Input: part model. Units: mm. Frame: model coordinates. Round coordinates to 2 decimals unless told otherwise and drop trailing zeros. Order: outer loops, then holes, each group sorted by start corner. A loop starts at its lowest first (then second) coordinate and runs counter-clockwise, first axis right, second up. Notation, with made-up numbers: (0.25, 64.25) - (9.25, 64.25) arc R11 ccw to (9.25, 80.25) - close; hole circle Ø4 at (79, 1.5). An arc over 180 degrees is marked (long way). One line per item, written item: value. Start each with the question number.
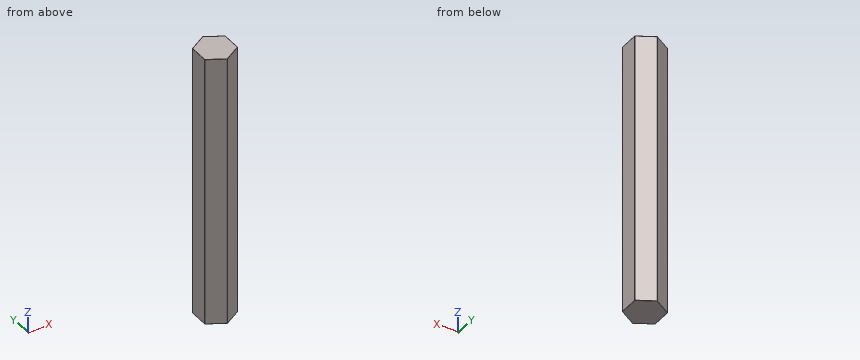
from build123d import *

# Parameters (mm, degrees)
F1_DEPTH = 200
F2_R     = 0.2


with BuildPart() as f1:
    # F0 (on Top) → F1 (new body)
    with BuildSketch(Plane.XY):
        Polygon((-0.015583, -13.856398), (11.992201, -6.941694), (12.007784, 6.914704), (0.015583, 13.856398), (-11.992201, 6.941694), (-12.007784, -6.914704), align=None)
    extrude(amount=F1_DEPTH)

    # F2
    f2_edges = [f1.edges().sort_by_distance(p)[0] for p in [
        (5.988309, -10.399046, 200),
        (11.999992, -0.013495, 200),
        (6.011683, 10.385551, 200),
        (-5.988309, 10.399046, 200),
        (-11.999992, 0.013495, 200),
        (-6.011683, -10.385551, 200),
        (11.992201, -6.941694, 100),
        (12.007784, 6.914704, 100),
        (11.999992, -0.013495, 0),
        (0.015583, 13.856398, 100),
        (6.011683, 10.385551, 0),
        (-11.992201, 6.941694, 100),
        (-5.988309, 10.399046, 0),
        (-12.007784, -6.914704, 100),
        (-11.999992, 0.013495, 0),
        (-0.015583, -13.856398, 100),
        (-6.011683, -10.385551, 0),
    ]]
    fillet(f2_edges, radius=F2_R)


solid = f1.part
Item 1: Line query: L1, parallel to X at y = -4.75, z = 93; L2, parallel to Y at x = 3.5, z = 164.5; L3, parallel to Y at x = 3.25, z = 119.5. Output: solid intervals per line, ascending.
Item 2: First-contact query: pin 1 Ø2 at (x, z) = (-5, 131) entering from +Y; pin 2 Ø4 at (x, z) = (-1.5, 29.5) entering from -Y; pin 3 Ø6 at (x, z) = (5, 135) entering from -Y; pin 4 Ø1 at (y, z) = (7, 103.5) entering from -X. Flat tips, straight axial feed; report the tip coordinate or a pass-through.
Item 3: Section query A-A on z = 119. Return loops of the section in (x, y).
Geometry results:
1. L1: x = -12.01 to 11.99
1. L2: y = -11.83 to 11.84
1. L3: y = -11.98 to 11.98
2. pin 1: stops at y = 11.54
2. pin 2: stops at y = -13.83
2. pin 3: stops at y = -12.7
2. pin 4: stops at x = -11.99
3. outline: (-12.01, -6.8) arc R0.2 ccw to (-11.91, -6.97) - (-0.12, -13.8) arc R0.2 ccw to (0.08, -13.8) - (11.89, -7) arc R0.2 ccw to (11.99, -6.83) - (12.01, 6.8) arc R0.2 ccw to (11.91, 6.97) - (0.12, 13.8) arc R0.2 ccw to (-0.08, 13.8) - (-11.89, 7) arc R0.2 ccw to (-11.99, 6.83) - close
